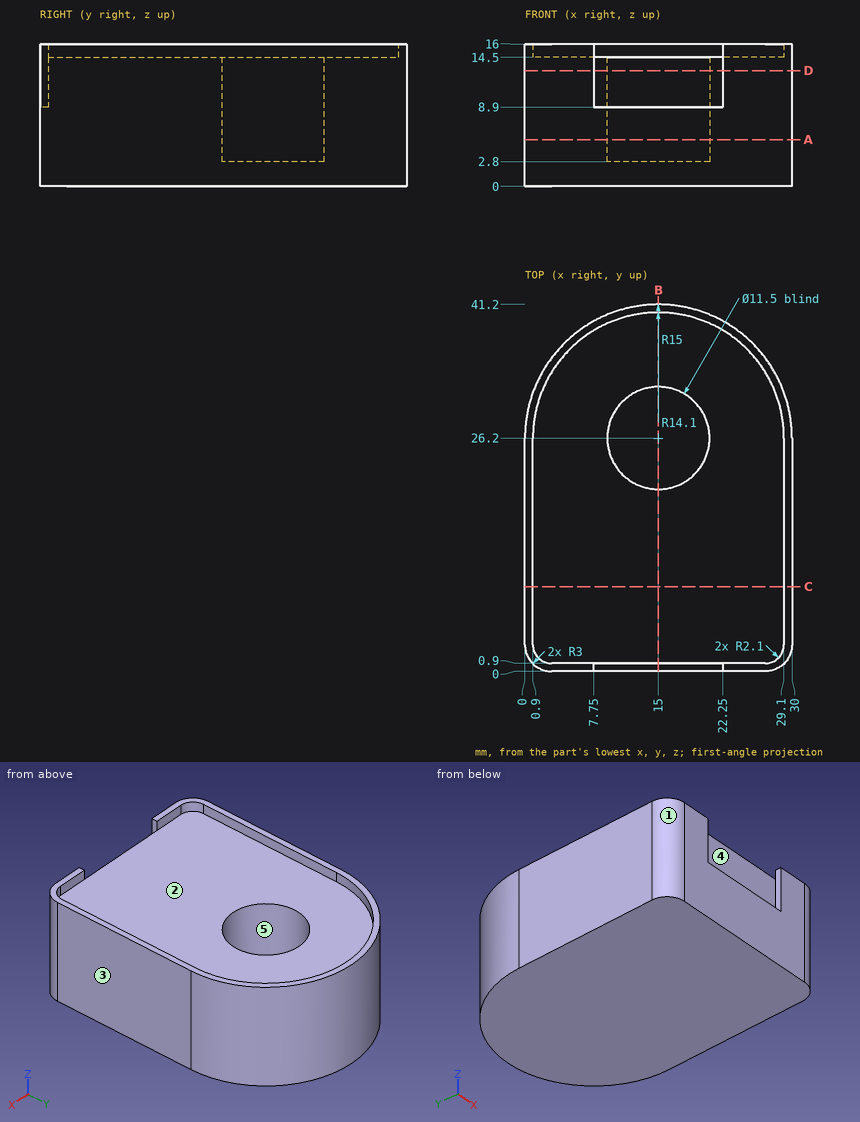
Part print with two shaded views. Sizes in mm from the minimum x, y, z corner. A direction names the side the tool comes from. Give positions to 0.01 mm unless a question says otherwise; leave off trailing zeros. Order: outer loops, then holes, each group sorted by start corner. A loop starts at its lowest first (then second) coordinate and runs counter-clockwise, first axis right, second up. Notation, with made-up numbers: M -20,64 L 19,64 A21 cw 19,74 Z; hole C 31,-23.5 d5. An arc over 180 degrees is marked long. Put each result on its own line as item: value.
Item 1: Wall check: probe 1 along Y at (x, z) = (15, 5.5); probe 2 along Y at (x, z) = (15, 11.25); probe 3 along Z at (x, y) = (27.75, 6.5). Give the ranges that are in metal, low to high.
Results are:
probe 1: 0 to 20.45, 31.95 to 41.2
probe 2: 0.9 to 20.45, 31.95 to 41.2
probe 3: 0 to 14.5
Item 2: Drop flat-ended pins along their axis: pin 1 Ø10 at (x, y) = (19.5, 37) entering from +Z; pin 2 Ø8 at (x, z) = (21, 9.5) entering from +Y; pin 3 Ø14 at (x, y) = (20, 25) entering from +Z; pin 4 Ø1.2 at (x, z) = (25.5, 15) entering from +Y. Give the stop position or say it passes through.
Results are:
pin 1: z = 16
pin 2: y = 41.07
pin 3: z = 14.5
pin 4: y = 37.47
Item 3: Cut at B-B on x = 15. Write the cut outline in (y, z).
Results are:
outline: M 0,0 L 41.2,0 L 41.2,16 L 40.3,16 L 40.3,14.5 L 31.95,14.5 L 31.95,2.8 L 20.45,2.8 L 20.45,14.5 L 0.9,14.5 L 0.9,8.9 L 0,8.9 Z
Item 4: Pull direction Y, two halves, no side cores. Call the marked faces 3, 4 and 5: +Y half, -Y half, draft (parallel to the pull), parting line (faces both ways), or undercut.
Results are:
face 3: draft
face 4: -Y half
face 5: undercut
Item 5: Cut at C-C on y = 9.5. Write the cut outline in (x, z).
Results are:
outline: M 0,0 L 30,0 L 30,16 L 29.1,16 L 29.1,14.5 L 0.9,14.5 L 0.9,16 L 0,16 Z
Item 6: Which spindle directions (+Z, -Z, +X, -X, +Y, -Y) get a long thin tool onto all of the face, cutting with end or side? Do the marked faces 1 and 2. Say none if no direction does.
Results are:
face 1: +Z, -Z, -X, -Y
face 2: +Z
Item 7: Cut at D-D on z = 13. Write the cut outline in (x, y).
Results are:
outline: M 0,3 A3 ccw 3,0 L 7.75,0 L 7.75,0.9 L 22.25,0.9 L 22.25,0 L 27,0 A3 ccw 30,3 L 30,26.2 A15 ccw 0,26.2 Z; hole C 15,26.2 d11.5
Item 8: Cut at A-A on z = 5.25. Write the cut outline in (x, y), then the cut area to 3 significant figures.
Results are:
outline: M 0,3 A3 ccw 3,0 L 27,0 A3 ccw 30,3 L 30,26.2 A15 ccw 0,26.2 Z; hole C 15,26.2 d11.5
area: 1,030 mm2
